Part model, mm, in its own coordinate system. A direction names the side the tool comes from. Coordinates: 2 decimals unless noted, no trailing zeros. Loops run counter-clockwise (first coordinate to the right, second up) from the corner with the lowest first, then second, coordinate; pieces in that order, holes last. Notation, with made-up numbers: M -37,23.25 L -17,23.25 A25 ccw -17,45.25 Z; hole C 0,-19 d9. An arc over 180 degrees is marked long. Use a Markdown table: item, result. Add a question column.
1) Pin check, flat tips, straight feed: pin 1 Ø1 at (x, y) = (-7.5, -20.5) entering from -Z; pin 2 Ø2.5 at (y, z) = (-5.5, 6) entering from +X; pin 3 Ø5.5 at (y, z) = (-29.5, 36) entering from -X; pin 4 Ø3 at (x, y) = (3.13, 19.79) entering from +Z. Stop position of each tip, or through.
2) Band-saw the part on D-D (z = 43). List the corners of the cut face in (x, y) (3 decimals), plus the area to 3 significant figures.
3) Tool access for faces 1 (the cylindrical face through (-2.31, -24.03, 35.08)), 2 (the flat face through (3, 13.436, 35)), 3 (the flat face through (-39.728, 19, 35)), 4 (the cylindrical face through (-24.474, -3.576, 87.009)): list every direction of +Z, -Z, +X, -X, +Y, -Y with a clear straight run to the whole face (end or side of a thin tool).
4) Band-saw the part on C-C (y = -18). List the corners of the cut face in (x, z).
5) Pull direction Y, two halves, no side cores. Call faces 5 (the cylindrical face through (3.568, 21.738, 72.198)), 6 (the flat face through (2, -23.077, 35)), 7 (the cylindrical face through (-48.347, 22.006, 72.198)): released by +Y, released by -Y, zero draft, split by the parting line, or undercut.
6) Wall check: probe 1 along Z at (x, y) = (-25, 10.5); probe 2 along X at (y, z) = (-8, 33.5); probe 3 along Z at (x, y) = (-41, -26.5). Give the ranges that are in metal, low to high. Write a range as from..to.
7) Band-saw the part on A-A (z = 73). List the corners of the cut face in (x, y) (3 decimals).
8) Band-saw the part on B-B (x = -8.5). List the corners of the cut face in (y, z).
from build123d import *

# Parameters (mm, degrees)
BOSS_EXTRUDE1_DEPTH = 69.85
SKETCH2_R           = 2
BOSS_EXTRUDE2_DEPTH = 4.7625
SKETCH3_R           = 3.25
BOSS_EXTRUDE3_DEPTH = 25.4
FILLET1_R           = 1.27
FILLET2_R           = 0.254
SKETCH4_R           = 0.80002704
SKETCH4_R_2         = 0.877357611
SKETCH4_R_3         = 0.997824801
SKETCH4_R_4         = 0.748045891
BOSS_EXTRUDE4_DEPTH = 12.7
CUT_EXTRUDE1_DEPTH  = 12.7
SKETCH6_W           = 4.683113718
SKETCH6_H           = 5.652977511
BOSS_EXTRUDE5_DEPTH = 1.5875


with BuildPart() as part:
    # Sketch1 → Boss-Extrude1 (new body)
    with BuildSketch(Plane.XY):
        with BuildLine():
            Line((-39.727633427, -26.251720506), (-39.727633427, -31.331720506))
            ThreePointArc((-39.727633427, -31.331720506), (-39.355659039, -32.229746118), (-38.457633427, -32.601720506))
            Line((-38.457633427, -32.601720506), (-4.485133427, -32.601720506))
            ThreePointArc((-4.485133427, -32.601720506), (-3.587107815, -32.229746118), (-3.215133427, -31.331720506))
            Line((-3.215133427, -31.331720506), (-3.215133427, -26.251720506))
            ThreePointArc((-3.215133427, -26.251720506), (-2.285197457, -24.006656475), (-0.040133427, -23.076720506))
            Line((-0.040133427, -23.076720506), (5.039866573, -23.076720506))
            ThreePointArc((5.039866573, -23.076720506), (5.937892185, -22.704746118), (6.309866573, -21.806720506))
            Line((6.309866573, -21.806720506), (6.309866573, 12.165779494))
            ThreePointArc((6.309866573, 12.165779494), (5.937892185, 13.063805106), (5.039866573, 13.435779494))
            Line((5.039866573, 13.435779494), (-0.040133427, 13.435779494))
            ThreePointArc((-0.040133427, 13.435779494), (-2.285197457, 14.365715464), (-3.215133427, 16.610779494))
            Line((-3.215133427, 16.610779494), (-3.215133427, 21.690779494))
            ThreePointArc((-3.215133427, 21.690779494), (-3.587107815, 22.588805106), (-4.485133427, 22.960779494))
            Line((-4.485133427, 22.960779494), (-38.457633427, 22.960779494))
            ThreePointArc((-38.457633427, 22.960779494), (-39.355659039, 22.588805106), (-39.727633427, 21.690779494))
            Line((-39.727633427, 21.690779494), (-39.727633427, 16.610779494))
            ThreePointArc((-39.727633427, 16.610779494), (-40.657569397, 14.365715464), (-42.902633427, 13.435779494))
            Line((-42.902633427, 13.435779494), (-47.982633427, 13.435779494))
            ThreePointArc((-47.982633427, 13.435779494), (-48.880659039, 13.063805106), (-49.252633427, 12.165779494))
            Line((-49.252633427, 12.165779494), (-49.252633427, -21.806720506))
            ThreePointArc((-49.252633427, -21.806720506), (-48.880659039, -22.704746118), (-47.982633427, -23.076720506))
            Line((-47.982633427, -23.076720506), (-42.902633427, -23.076720506))
            ThreePointArc((-42.902633427, -23.076720506), (-40.657569397, -24.006656475), (-39.727633427, -26.251720506))
        make_face()
    extrude(amount=BOSS_EXTRUDE1_DEPTH)

    # Sketch2 → Boss-Extrude2 (add)
    with BuildSketch(Plane.XY.offset(69.85)):
        with BuildLine():
            Line((-46.077633427, 22.960779494), (3.134866573, 22.960779494))
            ThreePointArc((3.134866573, 22.960779494), (5.379930603, 22.030843525), (6.309866573, 19.785779494))
            Line((6.309866573, 19.785779494), (6.309866573, -29.426720506))
            ThreePointArc((6.309866573, -29.426720506), (5.379930603, -31.671784536), (3.134866573, -32.601720506))
            Line((3.134866573, -32.601720506), (-46.077633427, -32.601720506))
            ThreePointArc((-46.077633427, -32.601720506), (-48.322697457, -31.671784536), (-49.252633427, -29.426720506))
            Line((-49.252633427, -29.426720506), (-49.252633427, 19.785779494))
            ThreePointArc((-49.252633427, 19.785779494), (-48.322697457, 22.030843525), (-46.077633427, 22.960779494))
        make_face()
        with Locations(Location((-46.077633427, 19.785779494, 0), (0, 0, 180))):
            Circle(SKETCH2_R, mode=Mode.SUBTRACT)
        with Locations(Location((3.134866573, 19.785779494, 0), (0, 0, 180))):
            Circle(SKETCH2_R, mode=Mode.SUBTRACT)
        with Locations(Location((3.134866573, -29.426720506, 0), (0, 0, 180))):
            Circle(SKETCH2_R, mode=Mode.SUBTRACT)
        with Locations(Location((-46.077633427, -29.426720506, 0), (0, 0, 180))):
            Circle(SKETCH2_R, mode=Mode.SUBTRACT)
    extrude(amount=BOSS_EXTRUDE2_DEPTH)

    # Sketch3 → Boss-Extrude3 (add)
    with BuildSketch(Plane.XY.offset(74.6125)):
        with Locations(Location((-21.471383427, -4.820470506, 0), (0, 0, 180))):
            Circle(SKETCH3_R)
    extrude(amount=BOSS_EXTRUDE3_DEPTH)

    # Fillet1
    fillet1_edges = [part.edges().sort_by_distance(p)[0] for p in [
        (-45.442633427, -23.076720506, 0),
        (-48.880659039, -22.704746118, 0),
        (-49.252633427, -4.820470506, 0),
        (-48.880659039, 13.063805106, 0),
        (-45.442633427, 13.435779494, 0),
        (-40.657569397, 14.365715464, 0),
        (-39.727633427, 19.150779494, 0),
        (-39.355659039, 22.588805106, 0),
        (-21.471383427, 22.960779494, 0),
        (-3.587107815, 22.588805106, 0),
        (-3.215133427, 19.150779494, 0),
        (-2.285197457, 14.365715464, 0),
        (2.499866573, 13.435779494, 0),
        (5.937892185, 13.063805106, 0),
        (6.309866573, -4.820470506, 0),
        (5.937892185, -22.704746118, 0),
        (2.499866573, -23.076720506, 0),
        (-2.285197457, -24.006656475, 0),
        (-3.215133427, -28.791720506, 0),
        (-3.587107815, -32.229746118, 0),
        (-21.471383427, -32.601720506, 0),
        (-39.355659039, -32.229746118, 0),
        (-39.727633427, -28.791720506, 0),
        (-40.657569397, -24.006656475, 0),
    ]]
    fillet(fillet1_edges, radius=FILLET1_R)

    # Fillet2
    fillet2_edges = [part.edges().sort_by_distance(p)[0] for p in [
        (-18.221383427, -4.820470506, 100.0125),
    ]]
    fillet(fillet2_edges, radius=FILLET2_R)

    # Sketch4 → Boss-Extrude4 (add)
    with BuildSketch(Plane(origin=(6.309866573, 0, 0), x_dir=(0, 0, -1), z_dir=(1, 0, 0))):
        with Locations(Location((-7.9375, -3.709220506, 0), (0, 0, 270))):
            Circle(SKETCH4_R)
        with Locations(Location((-5.715, -3.709220506, 0), (0, 0, 270))):
            Circle(SKETCH4_R_2)
        with Locations(Location((-7.9375, -5.931720506, 0), (0, 0, 270))):
            Circle(SKETCH4_R_3)
        with Locations(Location((-5.715, -5.931720506, 0), (0, 0, 270))):
            Circle(SKETCH4_R_4)
    extrude(amount=BOSS_EXTRUDE4_DEPTH)

    # Sketch5 → Cut-Extrude1 (cut)
    with BuildSketch(Plane(origin=(0, 0, 0), x_dir=(1, 0, 0), z_dir=(0, 1, 0))):
        with BuildLine():
            Line((19.40157432, -15.483292253), (15.569046376, -8.549651145))
            ThreePointArc((15.569046376, -8.549651145), (15.552114593, -8.341430664), (15.697013921, -8.190942663))
            Line((15.697013921, -8.190942663), (16.262546188, -7.964729756))
            ThreePointArc((16.262546188, -7.964729756), (16.409544972, -7.808110678), (16.383956807, -7.594842245))
            Line((16.383956807, -7.594842245), (15.425992047, -6.05311771))
            ThreePointArc((15.425992047, -6.05311771), (15.404972946, -5.827088801), (15.573063537, -5.674522674))
            Line((15.573063537, -5.674522674), (17.830264536, -5.040651161))
            ThreePointArc((17.830264536, -5.040651161), (18.003893911, -4.872306809), (17.957864643, -4.634886744))
            Line((17.957864643, -4.634886744), (14.477857706, -0.398356559))
            Line((14.477857706, -0.398356559), (15.904974427, 0.453519903))
            Line((15.904974427, 0.453519903), (25.632541799, -10.775224085))
            Line((25.632541799, -10.775224085), (19.40157432, -15.483292253))
        make_face()
    extrude(amount=-CUT_EXTRUDE1_DEPTH, mode=Mode.SUBTRACT)

    # Sketch6 → Boss-Extrude5 (add)
    with BuildSketch(Plane(origin=(6.309866573, 0, 0), x_dir=(0, 0, -1), z_dir=(1, 0, 0))):
        with Locations((-6.830267964, -4.820470506)):
            Rectangle(SKETCH6_W, SKETCH6_H)
    extrude(amount=BOSS_EXTRUDE5_DEPTH)


solid = part.part
Entries:
| question | item | result |
|---|---|---|
| 1 | pin 1 | z = 0 |
| 1 | pin 2 | x = 17.95 |
| 1 | pin 3 | x = -39.73 |
| 1 | pin 4 | through |
| 2 | outline | M -49.253,-21.807 A1.27 ccw -47.983,-23.077 L -42.903,-23.077 A3.175 cw -39.728,-26.252 L -39.728,-31.332 A1.27 ccw -38.458,-32.602 L -4.485,-32.602 A1.27 ccw -3.215,-31.332 L -3.215,-26.252 A3.175 cw -0.04,-23.077 L 5.04,-23.077 A1.27 ccw 6.31,-21.807 L 6.31,12.166 A1.27 ccw 5.04,13.436 L -0.04,13.436 A3.175 cw -3.215,16.611 L -3.215,21.691 A1.27 ccw -4.485,22.961 L -38.458,22.961 A1.27 ccw -39.728,21.691 L -39.728,16.611 A3.175 cw -42.903,13.436 L -47.983,13.436 A1.27 ccw -49.253,12.166 Z |
| 2 | area | 2,730 mm2 |
| 3 | face 1 | -Z, +X, -Y |
| 3 | face 2 | -Z, +X, +Y |
| 3 | face 3 | -Z, -X, +Y |
| 3 | face 4 | +Z |
| 4 | outline | M -49.25,1.27 A1.27 ccw -47.98,0 L 5.04,0 A1.27 ccw 6.31,1.27 L 6.31,74.61 L -49.25,74.61 Z |
| 5 | face 5 | undercut |
| 5 | face 6 | released by -Y |
| 5 | face 7 | released by +Y |
| 6 | probe 1 | 0..74.61 |
| 6 | probe 2 | -49.25..6.31 |
| 6 | probe 3 | 69.85..74.61 |
| 7 | outline | M -49.253,-29.427 A3.175 ccw -46.078,-32.602 L 3.135,-32.602 A3.175 ccw 6.31,-29.427 L 6.31,19.786 A3.175 ccw 3.135,22.961 L -46.078,22.961 A3.175 ccw -49.253,19.786 Z; hole C -46.078,-29.427 d4; hole C -46.078,19.786 d4; hole C 3.135,-29.427 d4; hole C 3.135,19.786 d4 |
| 8 | outline | M -32.6,1.27 A1.27 ccw -31.33,0 L 21.69,0 A1.27 ccw 22.96,1.27 L 22.96,74.61 L -32.6,74.61 Z |
